from build123d import *

# Parameters (mm, degrees)
SKETCH1_R           = 2.6
SKETCH1_R_2         = 6.9
BOSS_EXTRUDE1_DEPTH = 5
SKETCH2_R           = 2.6
SKETCH2_R_2         = 4
BOSS_EXTRUDE2_DEPTH = 2
SCALE1_SCALE        = 1.5


with BuildPart() as part:
    # Sketch1 → Boss-Extrude1 (new body)
    with BuildSketch(Plane.XY):
        with BuildLine():
            Line((-117.842377899, -77.068349263), (-91.221161774, -74.112086796))
            ThreePointArc((-91.221161774, -74.112086796), (-84.435913767, -76.1684327), (-78.267124508, -72.673552434))
            Line((-78.267124508, -72.673552434), (-21.451382857, -66.364214657))
            ThreePointArc((-21.451382857, -66.364214657), (-16.007105356, -59.559722092), (-22.811597922, -54.115444591))
            Line((-22.811597922, -54.115444591), (-79.542760834, -60.415389973))
            ThreePointArc((-79.542760834, -60.415389973), (-86.42258563, -58.278403776), (-92.665955577, -61.872709124))
            Line((-92.665955577, -61.872709124), (-119.079141177, -64.805869985))
            ThreePointArc((-119.079141177, -64.805869985), (-133.941604274, -72.498469269), (-117.842377899, -77.068349263))
        make_face()
        with Locations((-22.131490389, -60.239829624)):
            Circle(SKETCH1_R, mode=Mode.SUBTRACT)
        with Locations((-85.429249698, -67.223418238)):
            Circle(SKETCH1_R_2, mode=Mode.SUBTRACT)
        with Locations((-124.987033061, -71.595333402)):
            Circle(SKETCH1_R_2, mode=Mode.SUBTRACT)
    extrude(amount=BOSS_EXTRUDE1_DEPTH)

    # Sketch2 → Boss-Extrude2 (add)
    with BuildSketch(Plane.XY.offset(5)):
        with BuildLine():
            Line((-22.811597922, -54.115444591), (-79.542760834, -60.415389973))
            ThreePointArc((-79.542760834, -60.415389973), (-86.42258563, -58.278403776), (-92.665955577, -61.872709124))
            Line((-92.665955577, -61.872709124), (-119.079141177, -64.805869985))
            ThreePointArc((-119.079141177, -64.805869985), (-133.941604274, -72.498469269), (-117.842377899, -77.068349263))
            Line((-117.842377899, -77.068349263), (-91.221161774, -74.112086796))
            ThreePointArc((-91.221161774, -74.112086796), (-84.435913767, -76.1684327), (-78.267124508, -72.673552434))
            Line((-78.267124508, -72.673552434), (-21.451382857, -66.364214657))
            ThreePointArc((-21.451382857, -66.364214657), (-16.007105356, -59.559722092), (-22.811597922, -54.115444591))
        make_face()
        with Locations((-22.131490389, -60.239829624)):
            Circle(SKETCH2_R, mode=Mode.SUBTRACT)
        with Locations((-85.429249698, -67.223418238)):
            Circle(SKETCH2_R_2, mode=Mode.SUBTRACT)
        with Locations((-124.987033061, -71.595333402)):
            Circle(SKETCH2_R_2, mode=Mode.SUBTRACT)
    extrude(amount=BOSS_EXTRUDE2_DEPTH)


with BuildPart() as part_1:
    # Scale1: scaled about (-72.846730446, -65.862557014, 3.611202843)
    add(part.part.scale(SCALE1_SCALE).moved(Location((36.423365223, 32.931278507, -1.805601422))))


solid = part_1.part
Model file for the job. Use its own axes, mm. A direction names the side the tool comes from. Coordinates: 2 decimals unless noted, no trailing zeros. Order: outer loops, then holes, each group sorted by start corner. A loop starts at its lowest first (then second) coordinate and runs counter-clockwise, first axis right, second up. Notation, with made-up numbers: (15.25, 23.5) -> (35.25, 23.5) arc R30 ccw to (35.25, 49.5) -> close; hole circle Ø10 at (63, 30.5). An arc over 180 degrees is marked (long way). Return JSON: item names as keys, results as strings. Group by question number.
Item 1: Saw through at D-D on y = -51. Write the cut outline in (x, z), then the cut area to 3 significant figures.
Item 2: Flat gauge pins, fed straight in: P1, Ø7, axis at x = -151.06, y = -74.46, coming from the +Z side; P2, Ø1, axis at x = -137.5, z = 4, coming from the -Y side; P3, Ø1.5, axis at y = -61, z = 6.5, coming from the +X side; P4, Ø1.5, axis at x = -42, z = 6, coming from the +Y side. Where does each tip first touch, or does it go through?
Item 3: Saw through at C-C on x = -122.5. Write the cut outline in (y, z).
Item 4: Saw through at B-B on z = 3. Write the cut outline in (x, y), then the cut area to 3 significant figures.
Item 5: Wall check: line 1 along Y through (x, z) = (-150.5, 8); line 2 along X through (y, z) = (-58.5, 1.75); line 3 along X through (y, z) = (-76.5, 6.75). Give the ranges that are in metal, low to high. Write a range as [from, to].
Item 6: Pull direction Y, two halves, no side cores. Call faces 5 (the flat face through (-38.962, -71.413, 3.371)), 6 (the cylindrical face through (-93.06, -54.47, 3.37)), 7 (the flat face through (-70, -67, -1.806)), 8 (the cylindrical face through (-145.334, -72.659, 7.173)): pulls with the +Y half, pulls with the -Y half, needs draft (parallel to the pull), parting line crosses it, or undercut.
Item 7: Saw through at A-A on y = -72. Write the cut outline in (x, z), then the cut area to 3 significant figures.
Item 8: Tool access for faces 1 (the cylindrical face through (-93.02, -73.76, 7.17)), 2 (the flat face through (-39.75, -52.9, 3.37)), 3 (the flat face through (-120.654, -80.485, 3.371)), 4 (the cylindrical face through (-159.27, -80.76, 1.89)): list every direction of +Z, -Z, +X, -X, +Y, -Y with a clear straight run to the whole face (end or side of a thin tool).
Values found:
{
 "1": {"outline": "(-22.63, -1.81) -> (9.87, -1.81) -> (9.87, 8.69) -> (-22.63, 8.69) -> close", "area": "341 mm2"},
 "2": {"P1": "passes through", "P2": "stops at y = -82.41", "P3": "stops at x = 12.03", "P4": "stops at y = -53.07"},
 "3": {"outline": "(-80.69, -1.81) -> (-62.09, -1.81) -> (-62.09, 8.69) -> (-80.69, 8.69) -> close"},
 "4": {"outline": "(-142.2, -64.28) arc R13.5 ccw (long way) to (-140.34, -82.67) -> (-100.41, -78.24) arc R13.5 ccw to (-80.98, -76.08) -> (4.25, -66.62) arc R9.24 ccw to (2.21, -48.24) -> (-82.89, -57.69) arc R13.5 ccw to (-102.58, -59.88) -> close; hole circle Ø20.7 at (-151.06, -74.46); hole circle Ø20.7 at (-91.72, -67.9); hole circle Ø7.8 at (3.23, -57.43)", "area": "2,740 mm2"},
 "5": {"line 1": "y = [-87.95, -80.44], [-68.49, -60.97]", "line 2": "x = [-101.41, -96.04], [-87.4, -0.52], [6.98, 12.41]", "line 3": "x = [-164.4, -156.7], [-145.41, -81.31]"},
 "6": {"face 5": "pulls with the -Y half", "face 6": "pulls with the +Y half", "face 7": "needs draft", "face 8": "undercut"},
 "7": {"outline": "(-164.33, -1.81) -> (-161.11, -1.81) -> (-161.11, 5.69) -> (-156.53, 5.69) -> (-156.53, 8.69) -> (-164.33, 8.69) -> close; (-145.59, 5.69) -> (-141, 5.69) -> (-141, -1.81) -> (-101.23, -1.81) -> (-101.23, 5.69) -> (-96.1, 5.69) -> (-96.1, 8.69) -> (-145.59, 8.69) -> close; (-87.34, 5.69) -> (-82.22, 5.69) -> (-82.22, -1.81) -> (-44.25, -1.81) -> (-44.25, 8.69) -> (-87.34, 8.69) -> close", "area": "908 mm2"},
 "8": {"face 1": "+Z, -Z", "face 2": "+Z, -Z, +Y", "face 3": "+Z, -Z, -Y", "face 4": "-Z"}
}
